Input: part model. Units: mm. Frame: model coordinates. Face numbers are marked on the shaded views. A direction names the side the tool comes from. Round coordinates to 2 decimals unless told otherwise and drop trailing zeros. Order: outer loops, then holes, each group sorted by start corner. A loop starts at its lowest first (then second) coordinate and runs counter-clockwise, first axis right, second up. Notation, with made-up numbers: (37, 9.5) -> (67, 9.5) arc R19 cw to (67, 43.5) -> close; hole circle Ø11 at (68, 49.5). An arc over 180 degrees is marked (long way). Use a Markdown table: item, result.
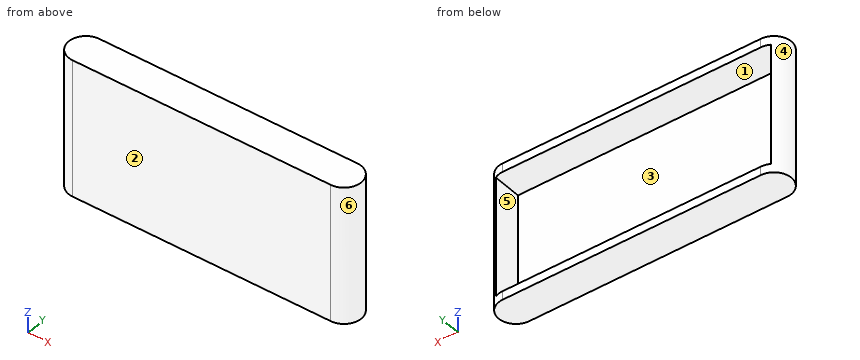
from build123d import *

# Parameters (mm, degrees)
BOSS_EXTRUDE1_DEPTH = 80
SKETCH2_W           = 159.903810567
SKETCH2_H           = 70
CUT_EXTRUDE1_DEPTH  = 18


with BuildPart() as part:
    # Sketch1 → Boss-Extrude1 (new body)
    with BuildSketch(Plane.XY):
        with BuildLine():
            Line((-3.900533574, 10.886474949), (126.003276993, 10.886474949))
            ThreePointArc((126.003276993, 10.886474949), (136.003276993, 0.886474949), (126.003276993, -9.113525051))
            Line((126.003276993, -9.113525051), (-3.900533574, -9.113525051))
            Line((-3.900533574, -9.113525051), (-23.900533574, -9.113525051))
            ThreePointArc((-23.900533574, -9.113525051), (-33.900533574, 0.886474949), (-23.900533574, 10.886474949))
            Line((-23.900533574, 10.886474949), (-3.900533574, 10.886474949))
        make_face()
    extrude(amount=-BOSS_EXTRUDE1_DEPTH)

    # Sketch2 → Cut-Extrude1 (cut)
    with BuildSketch(Plane(origin=(0, 10.886474949, 0), x_dir=(1, 0, 0), z_dir=(0, 1, 0))):
        with Locations((51.05137171, 40)):
            Rectangle(SKETCH2_W, SKETCH2_H)
    extrude(amount=-CUT_EXTRUDE1_DEPTH, mode=Mode.SUBTRACT)


solid = part.part
1) Cut plane C-C on z = -59. Return loops of the section in (x, y), and give its area (3 significant figures).
Results found:
| item | result |
|---|---|
| outline | (-28.9, -7.11) -> (-28.9, 9.55) arc R10 ccw to (-23.9, -9.11) -> (126, -9.11) arc R10 ccw to (131, 9.55) -> (131, -7.11) -> close |
| area | 438 mm² |
2) Pin query (flat end, axial travel): pin 1 Ø4 at (y, z) = (-4, -13.5) entering from -X; pin 2 Ø10 at (x, z) = (61, -69.5) entering from +Y. Return the tip coordinate at first contact, or that it passes through.
Results found:
| item | result |
|---|---|
| pin 1 | stops at x = -33.47 |
| pin 2 | stops at y = -7.11 |
3) Set-up query: the marked faces 1 and 2. Return all of +Z, -Z, +X, -X, +Y, -Y with unobstructed straight access to the full face (end or side cutting, diameter ignored); none if empty.
Results found:
| item | result |
|---|---|
| face 1 | +Y |
| face 2 | +Z, -Z, +X, -X, -Y |
4) Cut plane D-D on y = -3.75. Return loops of the section in (x, z), and give its area (3 significant figures).
Results found:
| item | result |
|---|---|
| outline | (-32.76, -80) -> (134.86, -80) -> (134.86, 0) -> (-32.76, 0) -> close; hole (-28.9, -75) -> (131, -75) -> (131, -5) -> (-28.9, -5) -> close |
| area | 2,220 mm² |
5) Pull-direction query (X, two-part tool) for the marked faces 3, 4, 5 and 6; classes: +X half, -X half, draft (parallel to the pull), parting line (faces both ways), or undercut.
Results found:
| item | result |
|---|---|
| face 3 | undercut |
| face 4 | -X half |
| face 5 | undercut |
| face 6 | +X half |
6) Cut plane B-B on y = 6.75. Return loops of the section in (x, z).
Results found:
| item | result |
|---|---|
| outline | (-32, -80) -> (134.1, -80) -> (134.1, 0) -> (-32, 0) -> close; hole (-28.9, -75) -> (131, -75) -> (131, -5) -> (-28.9, -5) -> close |
7) Line query: L1, parallel to X at y = 0.5, z = -68; L2, parallel to Z at x = 79, y = 5; L3, parallel to Y at x = 77, z = -11. Output: solid intervals per line, ascending. Write a range as [from, to].
Results found:
| item | result |
|---|---|
| L1 | x = [-33.89, -28.9], [131, 136] |
| L2 | z = [-80, -75], [-5, 0] |
| L3 | y = [-9.11, -7.11] |
8) Cut plane A-A on x = -17. Return loops of the section in (y, z).
Results found:
| item | result |
|---|---|
| outline | (-9.11, -80) -> (10.89, -80) -> (10.89, -75) -> (-7.11, -75) -> (-7.11, -5) -> (10.89, -5) -> (10.89, 0) -> (-9.11, 0) -> close |
